from build123d import *

# Parameters (mm, degrees)
SKETCH1_R          = 23.6855
EXTRUDE1_DEPTH     = 95.123
CHAMFER1_SIZE      = 0.762
SKETCH6_R          = 17.4625
EXTRUDE2_DEPTH     = 5.969
SKETCH7_W          = 33.655
SKETCH7_H          = 10.31875
CUT_EXTRUDE4_DEPTH = 19.84248
HOLE1_D            = 4.7498
HOLE1_DEPTH        = 4.7498
CIRPATTERN1_COUNT  = 4
LPATTERN1_COUNT    = 2
LPATTERN1_PITCH    = 28.5496


with BuildPart() as part:
    # Sketch1 → Extrude1 (new body)
    with BuildSketch(Plane.XY):
        Circle(SKETCH1_R)
    extrude(amount=EXTRUDE1_DEPTH)

    # Sketch2 → Cut-Revolve1 (revolve, cut)
    with BuildSketch(Plane(origin=(0, 0, 0), x_dir=(1, 0, 0), z_dir=(0, 1, 0)), mode=Mode.PRIVATE) as cut_revolve1_sk:
        Polygon((23.6855, -95.123), (23.6855, -81.153), (22.4155, -82.423), (22.4155, -95.123), align=None)
    revolve(cut_revolve1_sk.sketch.rotate(Axis((0, 0, 0), (0, 0, 1)), 180), axis=Axis((0, 0, 0), (0, 0, 1)), mode=Mode.SUBTRACT)  # turned: the seam where the file's is

    # Sketch3 → Cut-Revolve2 (revolve, cut)
    with BuildSketch(Plane(origin=(0, 0, 0), x_dir=(1, 0, 0), z_dir=(0, 1, 0)), mode=Mode.PRIVATE) as cut_revolve2_sk:
        Polygon((22.4155, 0), (22.4155, -1.524), (23.6855, -2.794), (23.6855, 0), align=None)
    revolve(cut_revolve2_sk.sketch.rotate(Axis((0, 0, 0), (0, 0, -1)), 180), axis=Axis((0, 0, 0), (0, 0, -1)), mode=Mode.SUBTRACT)  # turned: the seam where the file's is

    # Chamfer1
    chamfer1_edges = [part.edges().sort_by_distance(p)[0] for p in [
        (22.4155, 0, 95.123),
    ]]
    chamfer(chamfer1_edges, length=CHAMFER1_SIZE)

    # S2D0002 → Cut-Revolve3 (revolve, cut)
    with BuildSketch(Plane(origin=(0, 0, 0), x_dir=(0, -1, 0), z_dir=(1, 0, 0)), mode=Mode.PRIVATE) as cut_revolve3_sk:
        Polygon((20.4597, -94.869), (23.7998, -94.869), (23.7998, -95.123), (14.2748, -95.123), (14.2748, -80.899), (19.2532, -80.899), (19.2532, -91.652393135), (19.917106865, -92.3163), align=None)
    cut_revolve3 = revolve(cut_revolve3_sk.sketch.rotate(Axis((0, -14.2748, 14.6685), (0, 0, -1)), 270), axis=Axis((0, -14.2748, 14.6685), (0, 0, -1)), mode=Mode.SUBTRACT)  # turned: the seam where the file's is

    # Sketch6 → Extrude2 (add)
    with BuildSketch(Plane(origin=(0, 0, 0), x_dir=(-1, 0, 0), z_dir=(0, 0, -1))):
        with Locations(Location((0, 0, 0), (0, 0, 180))):  # turned: the seam where the file's is
            Circle(SKETCH6_R)
    extrude(amount=EXTRUDE2_DEPTH)

    # Sketch7 → Revolve1 (revolve)
    with BuildSketch(Plane(origin=(0, 0, 0), x_dir=(0, 0, -1), z_dir=(1, 0, 0)), mode=Mode.PRIVATE) as revolve1_sk:
        with Locations((22.7965, -5.159375)):
            Rectangle(SKETCH7_W, SKETCH7_H)
    revolve(revolve1_sk.sketch.rotate(Axis((0, 0, 0), (0, 0, -1)), 90), axis=Axis((0, 0, 0), (0, 0, -1)))  # turned: the seam where the file's is

    # S2D0001 → Cut-Revolve5 (revolve, cut)
    with BuildSketch(Plane(origin=(0, 0, 0), x_dir=(1, 0, 0), z_dir=(0, 1, 0))):
        Polygon((3.2639, 37.688260017), (3.2639, 24.5618), (0, 24.5618), (0, 39.624), (4.3815, 39.624), align=None)
    revolve(axis=Axis((0, 0, 31.308359971), (0, 0, -1)), mode=Mode.SUBTRACT)

    # Sketch9 → Cut-Revolve6 (revolve, cut)
    with BuildSketch(Plane(origin=(0, 0, 0), x_dir=(0, -1, 0), z_dir=(1, 0, 0)), mode=Mode.PRIVATE) as cut_revolve6_sk:
        with BuildLine():
            Line((-10.31875, 32.2072), (-10.033, 32.9692))
            Line((-10.033, 32.9692), (-10.033, 38.608))
            ThreePointArc((-10.033, 38.608), (-9.932678675, 39.151796865), (-9.644922533, 39.624))
            Line((-9.644922533, 39.624), (-10.31875, 39.624))
            Line((-10.31875, 39.624), (-10.31875, 32.2072))
        make_face()
    revolve(cut_revolve6_sk.sketch.rotate(Axis((0, 0, -12.65936), (0, 0, -1)), 90), axis=Axis((0, 0, -12.65936), (0, 0, -1)), mode=Mode.SUBTRACT)  # turned: the seam where the file's is

    # Sketch13 → Cut-Extrude4 (cut, symmetric)
    with BuildSketch(Plane(origin=(0, 0, 0), x_dir=(1, 0, 0), z_dir=(0, 1, 0))):
        Polygon((8.5852, 39.624), (8.5852, 34.671), (10.033, 33.2232), (10.033, 39.624), align=None)
        Polygon((-8.5852, 39.624), (-8.5852, 34.671), (-10.033, 33.2232), (-10.033, 39.624), align=None)
    extrude(amount=CUT_EXTRUDE4_DEPTH, both=True, mode=Mode.SUBTRACT)

    # Hole1
    with Locations(Plane(origin=(-15.850152054, 15.850152054, 88.773), x_dir=(0.707106781, 0.707106781, 0), z_dir=(-0.707106781, 0.707106781, 0))):
        with Locations((0, 0)):
            hole1 = Hole(HOLE1_D / 2, depth=HOLE1_DEPTH)

    # CirPattern1: Hole1 ×4 about axis
    cirpattern1_axis = Axis((0, 0, 0), (0, 0, 1))
    for i in range(1, CIRPATTERN1_COUNT):
        add(hole1.rotate(cirpattern1_axis, i * 360 / CIRPATTERN1_COUNT), mode=Mode.SUBTRACT)

    # LPattern1: Cut-Revolve3 ×2
    with Locations(*[(0, i * LPATTERN1_PITCH, 0) for i in range(1, LPATTERN1_COUNT)]):
        add(cut_revolve3, mode=Mode.SUBTRACT)


solid = part.part
Geometry check sheet. Reference: the model listing, model coordinates, mm. A direction names the side the tool comes from. Give positions to 0.01 mm unless a question says otherwise; leave off trailing zeros. Write each loop counter-clockwise with the first axis right and the second up, starting at its lowest first coordinate (ties: lowest second). Pieces come first, ordered by that corner, then holes.
1) Thickness scan on line 1 (Y direction, x = 0, z = 88.5); line 2 (Z direction, x = 0.5, y = 7.5); line 3 (Z direction, x = -7, y = -9.5). Record the ranges inside material, lowest first.
Values follow:
line 1: y = -22.42 to -19.25, -9.3 to 9.3, 19.25 to 22.42
line 2: z = -39.62 to 94.87
line 3: z = -5.97 to 94.87
2) Cross-section at B-B (z = 84.5). Record the boundary of the cut face in (x, y).
Values follow:
outline: circle Ø44.83 at (0, 0); hole circle Ø9.96 at (0, -14.27); hole circle Ø9.96 at (0, 14.27)
3) Go/stop test with flat-tipped pins: pin 1 Ø5 at (x, y) = (-0.5, 14) entering from +Z; pin 2 Ø1.5 at (x, z) = (-16.5, 22.5) entering from -Y; pin 3 Ø13.5 at (x, y) = (4.5, 9.5) entering from +Z; pin 4 Ø4 at (y, z) = (3, 40) entering from -X. Record where each tip stops, or that it passes through.
Values follow:
pin 1: stops at z = 80.9
pin 2: stops at y = -17.69
pin 3: stops at z = 95.12
pin 4: stops at x = -23.66
4) Release check for a two-part mould opening along Y. For faces 1 (the face through (-14.51, -13.78, 91.09)), 2 (the face through (8.585, 0, -37)), 3 (the face through (-20.7, 8.6, 88.5)) record: released by +Y, released by -Y, zero draft, split by the parting line, or undercut.
Values follow:
face 1: undercut
face 2: zero draft
face 3: split by the parting line
5) Cross-section at A-A (z = -9). Record the boundary of the cut face in (x, y), plus the area to 3 significant figures.
Values follow:
outline: circle Ø20.64 at (0, 0)
area: 335 mm2
6) Set-up check for faces 4 (the face through (-8.585, 0, -37)), 5 (the face through (14.51, 13.78, 91.09)), 6 (the face through (-1.079, -9.415, 86.351)), 7 (the face through (-0.708, 3.186, -31.033)): record each of +Z, -Z, +X, -X, +Y, -Y from which the full face is reachable in a straight line by a thin tool's end or side.
Values follow:
face 4: -Z, -X, +Y, -Y
face 5: none
face 6: +Z
face 7: -Z
